Autodesk Inventor part; units mm, degrees
ref_plane "YZ Plane" through (0, 0, 0) normal (1, 0, 0) x (0, 1, 0)
ref_plane "XZ Plane" through (0, 0, 0) normal (0, 1, 0) x (-1, 0, 0)
ref_plane "XY Plane" through (0, 0, 0) normal (0, 0, 1) x (1, 0, 0)
sketch "Эскиз1" plane through (0, 0, 0) normal (0, 1, 0) x (-1, 0, 0)
  line L0 (0, 0) -> (-220, 0)
  line L1 (-220, 0) -> (-220, -30)
  line L2 (-220, -30) -> (0, -30)
  line L3 (0, -30) -> (0, 0)
  dimension "d0" = 220
  dimension "d1" = 30
extrude "Выдавливание1" add sketch "Эскиз1" along normal blind 80
chamfer "Фаска1" distance 30 angle 45 2 edges at (0, 40, 0) (220, 40, 0)
properties part number "dou_long" material "Красное дерево"
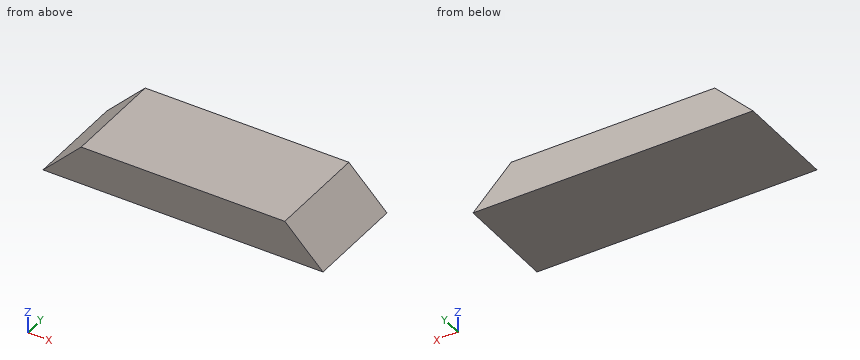
Model file for the job. Use its own axes, mm. Give positions to 0.01 mm unless a question says otherwise; leave off trailing zeros. Loops run counter-clockwise (first coordinate to the right, second up) from the corner with the lowest first, then second, coordinate; pieces in that order, holes last. Notation, with made-up numbers: (-9.5, 55) -> (42.5, 55) arc R21 ccw to (42.5, 78) -> close; hole circle Ø11 at (82.25, 54). An arc over 180 degrees is marked (long way). Use a Markdown table: item, result. Add a question column.
(1) Slice it at B-B on z = -9.75. List the corners of the cut face in (x, y), and give its area (3 significant figures).
(2) Slice it at C-C on x = 22. List the corners of the cut face in (y, z).
(3) Wall check: line 1 along X through (y, z) = (12, -26.5); line 2 along Z through (x, y) = (210, 71.5); line 3 along X through (y, z) = (59, -7.25). Give the ranges that are in metal, low to high.
(4) Drop flat-ended pins along their axis: pin 1 Ø1.5 at (x, z) = (183, -13) entering from -Y; pin 2 Ø12 at (y, z) = (26, -15) entering from -X. Give the stop position or say it passes through.
Filled sheet:
| question | item | result |
|---|---|---|
| 1 | outline | (20.25, 0) -> (199.75, 0) -> (199.75, 80) -> (20.25, 80) -> close |
| 1 | area | 14,400 mm2 |
| 2 | outline | (0, -30) -> (80, -30) -> (80, -8) -> (0, -8) -> close |
| 3 | line 1 | 3.5 to 216.5 |
| 3 | line 2 | -30 to -20 |
| 3 | line 3 | 22.75 to 197.25 |
| 4 | pin 1 | y = 0 |
| 4 | pin 2 | x = 9 |
